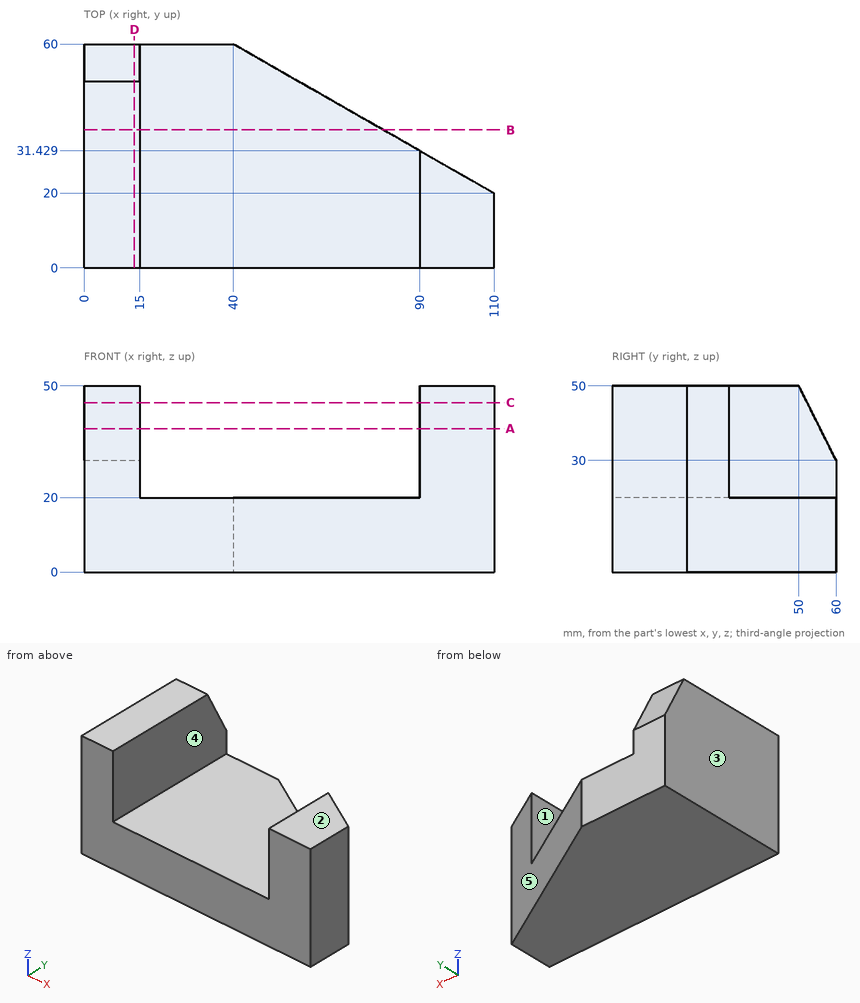
Input: dimensioned drawing with shaded views. Units: mm. Origin: part minimum x, y, z. A direction names the side the tool comes from. Round coordinates to 2 decimals unless told otherwise and drop trailing zeros. Order: outer loops, then holes, each group sorted by start corner. A loop starts at its lowest first (then second) coordinate and runs counter-clockwise, first axis right, second up. Notation, with made-up numbers: (29.5, 50) - (70.5, 50) arc R17 cw to (70.5, 56) - close; hole circle Ø11 at (-29.75, 19.5). An arc over 180 degrees is marked (long way). Write item = value, one per line. Start each with the question number.
Q1. Cut plane A-A on z = 38.5. Return the cut outline in (x, y).
Q2. Cut plane B-B on y = 37. Return the cut outline in (x, z), and give its area (4 significant figures).
Q3. Cut plane D-D on x = 13.5. Return the cut outline in (y, z).
Q4. Pin query (flat end, axial travel): pin 1 (6 mm diameter, centred on x = 26.5, y = 40, fed in from +Z); pin 2 (3 mm diameter, centred on x = 51.5, z = 5, fed in from +Y) (1 decimal); pin 3 (9 mm diameter, centred on y = 36.5, z = 39, fed in from +X); pin 4 (15 mm diameter, centred on y = 11, z = 42.5, fed in from -X). Return the tip coordinate at first contact, or that it passes through.
Q5. Cut plane C-C on z = 45.5. Return the cut outline in (x, y), and give its area (3 significant figures).
Q6. Access query for the marked faces 4 and 5. Directions: +Z, -Z, +X, -X, +Y, -Y. A direction counts if a zero-diameter tool reaches every point of the face in a straight line with its end or side. Return the directions, or none.
Q7. Ray query, line 1 (X direction, y = 33, z = 25); line 2 (Z direction, x = 55, y = 14); line 3 (X direction, y = 26.5, z = 46.5) (1 decimal). Return the intervals inside material, ascending. Write a range as from..to.
Q8. Pull-direction query (X, two-part tool) for the marked faces 1, 2 and 3; classes: +X half, -X half, draft (parallel to the pull), parting line (faces both ways), or undercut.
Outcome:
q1.outline = (0, 0) - (15, 0) - (15, 55.75) - (0, 55.75) - close; (90, 0) - (110, 0) - (110, 20) - (90, 31.43) - close
q2.outline = (0, 0) - (80.25, 0) - (80.25, 20) - (15, 20) - (15, 50) - (0, 50) - close
q2.area = 2,055 mm^2
q3.outline = (0, 0) - (60, 0) - (60, 30) - (50, 50) - (0, 50) - close
q4.pin_1 = 20
q4.pin_2 = 54.3
q4.pin_3 = 15
q4.pin_4 = 0
q5.outline = (0, 0) - (15, 0) - (15, 52.25) - (0, 52.25) - close; (90, 0) - (110, 0) - (110, 20) - (90, 31.43) - close
q5.area = 1,300 mm^2
q6.face_4 = +Z, +Y, -Y
q6.face_5 = +Z, -Z, +X, +Y
q7.line_1 = 0..15
q7.line_2 = 0..20
q7.line_3 = 0..15, 90..98.6
q8.face_1 = undercut
q8.face_2 = draft
q8.face_3 = -X half
